from build123d import *

# Parameters (mm, degrees)
SKETCH1_R                = 15.5
SKETCH1_R_2              = 13.5
BOSS_EXTRUDE1_DEPTH      = 4
CUT_EXTRUDE1_DEPTH       = 44
CUT_EXTRUDE1_DEPTH_BACK  = 44
CUT_EXTRUDE2_DEPTH       = 44
CUT_EXTRUDE2_DEPTH_BACK  = 44
BOSS_EXTRUDE2_DEPTH      = 1
BOSS_EXTRUDE2_DEPTH_BACK = 1
SKETCH5_R                = 1.5
CUT_EXTRUDE3_DEPTH       = 3
BOSS_EXTRUDE3_DEPTH      = 1.5
BOSS_EXTRUDE3_DEPTH_BACK = 3.5
SKETCH6_R                = 5.5
SKETCH6_R_2              = 1.5
SKETCH7_R                = 1.5
CUT_EXTRUDE4_DEPTH       = 11.5


with BuildPart() as part:
    # Sketch1 → Boss-Extrude1 (new body)
    with BuildSketch(Plane(origin=(0, 0, 0), x_dir=(1, 0, 0), z_dir=(0, 1, 0))):
        with Locations(Location((0, 0, 0), (0, 0, 270))):
            Circle(SKETCH1_R)
        with Locations(Location((0, 0, 0), (0, 0, 270))):
            Circle(SKETCH1_R_2, mode=Mode.SUBTRACT)
    extrude(amount=BOSS_EXTRUDE1_DEPTH)

    # Sketch2 → Cut-Extrude1 (cut, two sides: drawn at the far end of the back side and taken through both)
    with BuildSketch(Plane.XY.offset(-CUT_EXTRUDE1_DEPTH_BACK)):
        with BuildLine():
            Line((-3, 3), (3, 3))
            ThreePointArc((3, 3), (4, 2), (3, 1))
            Line((3, 1), (-3, 1))
            ThreePointArc((-3, 1), (-4, 2), (-3, 3))
        make_face()
    extrude(amount=CUT_EXTRUDE1_DEPTH + CUT_EXTRUDE1_DEPTH_BACK, mode=Mode.SUBTRACT)

    # Sketch3 → Cut-Extrude2 (cut, two sides: drawn at the far end of the back side and taken through both)
    with BuildSketch(Plane(origin=(0, 0, 0), x_dir=(0, 0, -1), z_dir=(1, 0, 0)).offset(-CUT_EXTRUDE2_DEPTH_BACK)):
        with BuildLine():
            Line((-3, 3), (3, 3))
            ThreePointArc((3, 3), (4, 2), (3, 1))
            Line((3, 1), (-3, 1))
            ThreePointArc((-3, 1), (-4, 2), (-3, 3))
        make_face()
    extrude(amount=CUT_EXTRUDE2_DEPTH + CUT_EXTRUDE2_DEPTH_BACK, mode=Mode.SUBTRACT)

    # Sketch4 → Boss-Extrude2 (add, two sides: drawn at the far end of the back side and taken through both)
    with BuildSketch(Plane(origin=(0, 2, 0), x_dir=(1, 0, 0), z_dir=(0, 1, 0)).offset(-BOSS_EXTRUDE2_DEPTH_BACK)):
        with BuildLine():
            Line((10.606601718, 15.556349186), (0, 4.949747468))
            Line((0, 4.949747468), (4.949747468, 0))
            Line((4.949747468, 0), (15.556349186, 10.606601718))
            ThreePointArc((15.556349186, 10.606601718), (15.556349186, 15.556349186), (10.606601718, 15.556349186))
        make_face()
        with BuildLine():
            Line((15.556349186, -10.606601718), (4.949747468, 0))
            Line((4.949747468, 0), (0, -4.949747468))
            Line((0, -4.949747468), (10.606601718, -15.556349186))
            ThreePointArc((10.606601718, -15.556349186), (15.556349186, -15.556349186), (15.556349186, -10.606601718))
        make_face()
        with BuildLine():
            Line((0, -4.949747468), (-4.949747468, 0))
            Line((-4.949747468, 0), (-15.556349186, -10.606601718))
            ThreePointArc((-15.556349186, -10.606601718), (-15.556349186, -15.556349186), (-10.606601718, -15.556349186))
            Line((-10.606601718, -15.556349186), (0, -4.949747468))
        make_face()
        Polygon((4.949747468, 0), (0, 4.949747468), (-4.949747468, 0), (0, -4.949747468), align=None)
        with BuildLine():
            Line((0, 4.949747468), (-10.606601718, 15.556349186))
            ThreePointArc((-10.606601718, 15.556349186), (-15.556349186, 15.556349186), (-15.556349186, 10.606601718))
            Line((-15.556349186, 10.606601718), (-4.949747468, 0))
            Line((-4.949747468, 0), (0, 4.949747468))
        make_face()
    extrude(amount=BOSS_EXTRUDE2_DEPTH + BOSS_EXTRUDE2_DEPTH_BACK)

    # Sketch5 → Cut-Extrude3 (cut)
    with BuildSketch(Plane(origin=(0, 3, 0), x_dir=(1, 0, 0), z_dir=(0, 1, 0))):
        with Locations(Location((0, 0, 0), (0, 0, 270))):
            Circle(SKETCH5_R)
    extrude(amount=-CUT_EXTRUDE3_DEPTH, mode=Mode.SUBTRACT)

    # Sketch6 → Boss-Extrude3 (add, two sides: drawn at the far end of the back side and taken through both)
    with BuildSketch(Plane(origin=(0, 3, 0), x_dir=(1, 0, 0), z_dir=(0, 1, 0)).offset(-BOSS_EXTRUDE3_DEPTH_BACK)):
        with Locations(Location((0, 0, 0), (0, 0, 270))):
            Circle(SKETCH6_R)
        with Locations(Location((0, 0, 0), (0, 0, 270))):
            Circle(SKETCH6_R_2, mode=Mode.SUBTRACT)
    extrude(amount=BOSS_EXTRUDE3_DEPTH + BOSS_EXTRUDE3_DEPTH_BACK)

    # Sketch7 → Cut-Extrude4 (cut)
    with BuildSketch(Plane(origin=(0, 3, 0), x_dir=(1, 0, 0), z_dir=(0, 1, 0))):
        with Locations(Location((-13.081475452, 13.081475452, 0), (0, 0, 270))):
            Circle(SKETCH7_R)
        with Locations(Location((13.081475452, 13.081475452, 0), (0, 0, 270))):
            Circle(SKETCH7_R)
        with Locations(Location((13.081475452, -13.081475452, 0), (0, 0, 270))):
            Circle(SKETCH7_R)
        with Locations(Location((-13.081475452, -13.081475452, 0), (0, 0, 270))):
            Circle(SKETCH7_R)
    extrude(amount=-CUT_EXTRUDE4_DEPTH, mode=Mode.SUBTRACT)


solid = part.part
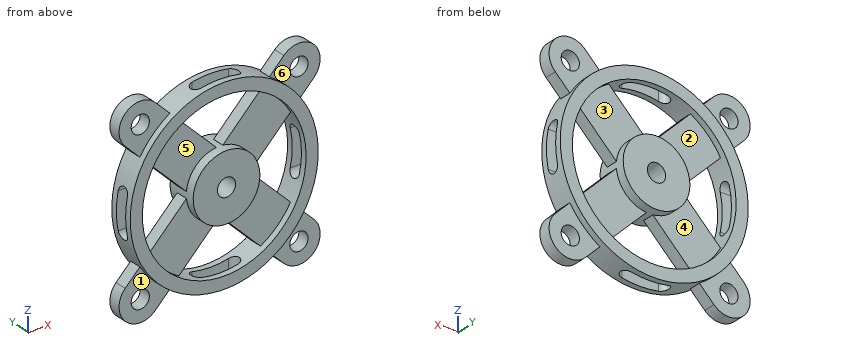
Build history of the part. All positions in model axes, mm. Face numbers are marked on the shaded views. A direction names the side the tool comes from. Round coordinates to 2 decimals unless told otherwise and drop trailing zeros. Loops run counter-clockwise (first coordinate to the right, second up) from the corner with the lowest first, then second, coordinate; pieces in that order, holes last. Notation, with made-up numbers: (41.5, 88.5) -> (97.5, 88.5) arc R26 cw to (97.5, 105.5) -> close; hole circle Ø7 at (-17, -8). An arc over 180 degrees is marked (long way). Answer in a Markdown table with one row per item.
Item 1: Drill centre lines: L1, parallel to X at y = 0.7, z = 0; L2, parallel to X at y = 1.6, z = 0; L3, parallel to Z at x = -3, y = 3.15. Where is each one in solid material? Low to high. Write a range as [from, to].
Answers below:
| item | result |
|---|---|
| L1 | x = [-15.5, -13.5], [-5.5, -1.5], [1.5, 5.5], [13.5, 15.5] |
| L2 | x = [-5.5, -1.5], [1.5, 5.5] |
| L3 | z = [-15.21, -13.16], [-4.61, 4.61], [13.16, 15.21] |
Item 2: Saw through at B-B (z = 10). Write the cut outline in (x, y), and give its area (3 significant figures).
Answers below:
| item | result |
|---|---|
| outline | (-14.95, 1) -> (-11.84, 1) -> (-11.84, 0) -> (-9.07, 0) -> (-9.07, 1) -> (-5.05, 1) -> (-5.05, 3) -> (-9.07, 3) -> (-9.07, 4) -> (-11.84, 4) -> (-11.84, 3) -> (-14.95, 3) -> close; (5.05, 1) -> (9.07, 1) -> (9.07, 0) -> (11.84, 0) -> (11.84, 1) -> (14.95, 1) -> (14.95, 3) -> (11.84, 3) -> (11.84, 4) -> (9.07, 4) -> (9.07, 3) -> (5.05, 3) -> close |
| area | 50.7 mm² |
Item 3: Saw through at A-A (x = 0). Write the cut outline in (y, z), and give its area (3 significant figures).
Answers below:
| item | result |
|---|---|
| outline | (-0.5, -5.5) -> (4.5, -5.5) -> (4.5, -1.5) -> (-0.5, -1.5) -> close; (-0.5, 1.5) -> (4.5, 1.5) -> (4.5, 5.5) -> (-0.5, 5.5) -> close; (0, -15.5) -> (1, -15.5) -> (1, -13.5) -> (0, -13.5) -> close; (0, 13.5) -> (1, 13.5) -> (1, 15.5) -> (0, 15.5) -> close; (3, -15.5) -> (4, -15.5) -> (4, -13.5) -> (3, -13.5) -> close; (3, 13.5) -> (4, 13.5) -> (4, 15.5) -> (3, 15.5) -> close |
| area | 48.0 mm² |
Item 4: Pin check, flat tips, straight feed: pin 1 (12.5 mm diameter, centred on x = 9, z = 6, fed in from +Y); pin 2 (4 mm diameter, centred on x = -10.5, z = -10.5, fed in from -Y); pin 3 (2.5 mm diameter, centred on x = 13.5, z = -11, fed in from +Y); pin 4 (2.5 mm diameter, centred on x = 1.5, z = 14.5, fed in from +Y). Stop position of each tip, or through.
Answers below:
| item | result |
|---|---|
| pin 1 | stops at y = 4.5 |
| pin 2 | stops at y = 0 |
| pin 3 | stops at y = 3 |
| pin 4 | stops at y = 4 |
Item 5: Saw through at C-C (z = -2). Write the cut outline in (x, y), and give its area (3 significant figures).
Answers below:
| item | result |
|---|---|
| outline | (-15.37, 0) -> (-13.35, 0) -> (-13.35, 1) -> (-15.37, 1) -> close; (-15.37, 3) -> (-13.35, 3) -> (-13.35, 4) -> (-15.37, 4) -> close; (-6.95, 1) -> (-5.12, 1) -> (-5.12, -0.5) -> (5.12, -0.5) -> (5.12, 1) -> (6.95, 1) -> (6.95, 3) -> (5.12, 3) -> (5.12, 4.5) -> (-5.12, 4.5) -> (-5.12, 3) -> (-6.95, 3) -> close; (13.35, 0) -> (15.37, 0) -> (15.37, 1) -> (13.35, 1) -> close; (13.35, 3) -> (15.37, 3) -> (15.37, 4) -> (13.35, 4) -> close |
| area | 66.6 mm² |
Item 6: Saw through at D-D (x = -10). Write the cut outline in (y, z).
Answers below:
| item | result |
|---|---|
| outline | (0, -11.84) -> (1, -11.84) -> (1, -14.95) -> (3, -14.95) -> (3, -11.84) -> (4, -11.84) -> (4, -9.07) -> (3, -9.07) -> (3, -5.05) -> (1, -5.05) -> (1, -9.07) -> (0, -9.07) -> close; (0, 9.07) -> (1, 9.07) -> (1, 5.05) -> (3, 5.05) -> (3, 9.07) -> (4, 9.07) -> (4, 11.84) -> (3, 11.84) -> (3, 14.95) -> (1, 14.95) -> (1, 11.84) -> (0, 11.84) -> close |
Item 7: Mould opens along Z. For the marked faces 1, 2 and 3 say: +Z half, -Z half, draft (parallel to the pull), parting line (faces both ways), or undercut.
Answers below:
| item | result |
|---|---|
| face 1 | draft |
| face 2 | undercut |
| face 3 | undercut |
Item 8: Which spindle directions (+Z, -Z, +X, -X, +Y, -Y) get a long thin tool onto all of the face, cutting with end or side? Do the marked faces 4, 5 and 6. Say none if no direction does.
Answers below:
| item | result |
|---|---|
| face 4 | +Y |
| face 5 | -Y |
| face 6 | +Z, +X, -Y |
